Design review of the part built by this model. Coordinates are the model's own, in mm. A direction names the side the tool comes from. Give positions to 0.01 mm unless a question says otherwise; leave off trailing zeros. Loops run counter-clockwise (first coordinate to the right, second up) from the corner with the lowest first, then second, coordinate; pieces in that order, holes last. Notation, with made-up numbers: (34.5, -26.5) -> (55.5, -26.5) arc R35 ccw to (55.5, 5.5) -> close; hole circle Ø10 at (12, 6.25). An arc over 180 degrees is marked (long way). Answer in a Markdown table with one row per item. Add a question column.
(1) Draft analysis for pull direction X (two halves, no side actions). For faces 1 (the flat face through (-25, 1, 25)), 2 (the flat face through (19.104, 55.481, -0.675)), state which applies: +X half, -X half, draft (parallel to the pull), parting line (faces both ways), or undercut.
(2) For faces 3 (the cylindrical face through (2.994, 22.804, -0.084)), 4 (the flat face through (33, -49, -12)), 5 (the flat face through (-46.86, 35.31, -0.68)), list the 3-axis set-ups (+Z, -Z, +X, -X, +Y, -Y) from which the entire face can be reached by the end or side of a thin tool; tool diameter is ignored.
(3) Consider section C-C on x = -58.5. Write out the cut boundary in (y, z).
(4) For line 1 (Y direction, x = 0, z = -11); line 2 (Y direction, x = -59.5, z = -12.5); line 3 (X direction, y = 20, z = -10), list the stretches that pass through material, from the lowest coordinate up.
(5) Consider section D-D on y = -68. Write out the cut boundary in (x, z).
(6) For pin 1 (2 mm diameter, centred on y = 52, z = 18.5, fed in from +X); pin 2 (1.5 mm diameter, centred on x = 6.5, z = -3.5, fed in from -Y); pin 3 (24 mm diameter, centred on x = 7.5, y = 66.5, fed in from +Z); pin 4 (3 mm diameter, centred on x = 30, y = 0, fed in from +Z), all flat-tipped, find the tip position at first contact; note any pin that passes through.
(7) Consider section A-A on z = -18. Write out the cut boundary in (x, y), then the cut area to 3 significant figures.
from build123d import *
from build123d.topology import SkipClean

# Parameters (mm, degrees)
SKETCH1_R           = 90
BOSS_EXTRUDE1_DEPTH = 25
SKETCH3_R           = 24
CUT_EXTRUDE2_DEPTH  = 19
CUT_EXTRUDE3_START  = -19
SKETCH4_R           = 24
CUT_EXTRUDE3_DEPTH  = 19
SKETCH5_R           = 23
CUT_EXTRUDE4_DEPTH  = 12
SKETCH6_R           = 82
SKETCH6_R_2         = 36
CUT_EXTRUDE7_DEPTH  = 12
CUT_EXTRUDE8_START  = -12
SKETCH8_R           = 82
SKETCH8_R_2         = 36
CUT_EXTRUDE8_DEPTH  = 12
CUT_EXTRUDE10_START = -25
CUT_EXTRUDE10_DEPTH = 25
CUT_EXTRUDE11_DEPTH = 25
SKETCH13_R          = 2
CUT_EXTRUDE12_DEPTH = 137.747943312


with BuildPart() as part:
    # Sketch1 → Boss-Extrude1 (new, symmetric)
    with BuildSketch(Plane.XY):
        Circle(SKETCH1_R)
    extrude(amount=BOSS_EXTRUDE1_DEPTH, both=True)

    # Sketch3 → Cut-Extrude2 (cut)
    with BuildSketch(Plane.XY.offset(25)):
        Circle(SKETCH3_R)
    extrude(amount=-CUT_EXTRUDE2_DEPTH, mode=Mode.SUBTRACT)

    # Sketch4 → Cut-Extrude3 (cut)
    with BuildSketch(Plane(origin=(0, 0, -25), x_dir=(-1, 0, 0), z_dir=(0, 0, -1)).offset(CUT_EXTRUDE3_START)):
        with Locations(Location((0, 0, 0), (0, 0, 180))):
            Circle(SKETCH4_R)
    extrude(amount=CUT_EXTRUDE3_DEPTH, mode=Mode.SUBTRACT)

    # Sketch5 → Cut-Extrude4 (cut)
    with BuildSketch(Plane(origin=(0, 0, -6), x_dir=(-1, 0, 0), z_dir=(0, 0, -1))):
        Circle(SKETCH5_R)
    extrude(amount=-CUT_EXTRUDE4_DEPTH, mode=Mode.SUBTRACT)

    # Sketch6 → Cut-Extrude7 (cut)
    with BuildSketch(Plane(origin=(0, 0, -25), x_dir=(-1, 0, 0), z_dir=(0, 0, -1))):
        Circle(SKETCH6_R)
        Circle(SKETCH6_R_2, mode=Mode.SUBTRACT)
    extrude(amount=-CUT_EXTRUDE7_DEPTH, mode=Mode.SUBTRACT)

    # Sketch8 → Cut-Extrude8 (cut)
    with BuildSketch(Plane.XY.offset(25).offset(CUT_EXTRUDE8_START)):
        with Locations(Location((0, 0, 0), (0, 0, 180))):
            Circle(SKETCH8_R)
        with Locations(Location((0, 0, 0), (0, 0, 180))):
            Circle(SKETCH8_R_2, mode=Mode.SUBTRACT)
    extrude(amount=CUT_EXTRUDE8_DEPTH, mode=Mode.SUBTRACT)

    # Sketch11 → Cut-Extrude10 (cut)
    with SkipClean():  # the faces are left unmerged after this step: merging them gives an invalid solid
        with BuildSketch(Plane.XY.offset(13).offset(CUT_EXTRUDE10_START)):
            with BuildLine():
                Line((11.124611797, 34.238034587), (25.339393539, 77.986634336))
                ThreePointArc((25.339393539, 77.986634336), (0, 82), (-25.339393539, 77.986634336))
                Line((-25.339393539, 77.986634336), (-11.124611798, 34.238034587))
                ThreePointArc((-11.124611798, 34.238034587), (0, 36), (11.124611797, 34.238034587))
            make_face()
            with BuildLine():
                Line((29.124611798, 21.160269083), (66.339393539, 48.198390688))
                ThreePointArc((66.339393539, 48.198390688), (77.986634336, 25.339393539), (82, 0))
                Line((82, 0), (36, 0))
                ThreePointArc((36, 0), (34.238034587, 11.124611797), (29.124611798, 21.160269083))
            make_face()
            with BuildLine():
                Line((29.124611798, -21.160269083), (66.339393539, -48.198390688))
                ThreePointArc((66.339393539, -48.198390688), (48.198390688, -66.339393539), (25.339393539, -77.986634336))
                Line((25.339393539, -77.986634336), (11.124611797, -34.238034587))
                ThreePointArc((11.124611797, -34.238034587), (21.160269083, -29.124611798), (29.124611798, -21.160269083))
            make_face()
            with BuildLine():
                Line((-11.124611797, -34.238034587), (-25.339393539, -77.986634336))
                ThreePointArc((-25.339393539, -77.986634336), (-48.198390688, -66.339393539), (-66.339393539, -48.198390688))
                Line((-66.339393539, -48.198390688), (-29.124611798, -21.160269083))
                ThreePointArc((-29.124611798, -21.160269083), (-21.160269083, -29.124611798), (-11.124611797, -34.238034587))
            make_face()
            with BuildLine():
                Line((-36, 0), (-82, 0))
                ThreePointArc((-82, 0), (-77.986634336, 25.339393539), (-66.339393539, 48.198390688))
                Line((-66.339393539, 48.198390688), (-29.124611798, 21.160269083))
                ThreePointArc((-29.124611798, 21.160269083), (-34.238034587, 11.124611797), (-36, 0))
            make_face()
        extrude(amount=CUT_EXTRUDE10_DEPTH, mode=Mode.SUBTRACT)

    # Sketch12 → Cut-Extrude11 (cut)
    with SkipClean():  # the faces are left unmerged after this step: merging them gives an invalid solid
        with BuildSketch(Plane(origin=(0, 0, -13), x_dir=(-1, 0, 0), z_dir=(0, 0, -1))):
            with BuildLine():
                ThreePointArc((-28.750878362, 21.665340833), (-21.160269083, 29.124611797), (-11.72045356, 34.038668722))
                Line((-11.72045356, 34.038668722), (-26.696588665, 77.532523199))
                ThreePointArc((-26.696588665, 77.532523199), (-48.198390688, 66.339393539), (-65.488111824, 49.348831898))
                Line((-65.488111824, 49.348831898), (-28.750878362, 21.665340833))
            make_face()
            with BuildLine():
                Line((26.696588665, 77.532523199), (11.72045356, 34.038668722))
                ThreePointArc((11.72045356, 34.038668722), (21.160269083, 29.124611797), (28.750878362, 21.665340833))
                Line((28.750878362, 21.665340833), (65.488111824, 49.348831898))
                ThreePointArc((65.488111824, 49.348831898), (48.198390688, 66.339393539), (26.696588665, 77.532523199))
            make_face()
            with BuildLine():
                Line((81.987511003, -1.431097328), (35.994517026, -0.628286632))
                ThreePointArc((35.994517026, -0.628286632), (34.238034587, -11.124611797), (29.489473594, -20.648751709))
                Line((29.489473594, -20.648751709), (67.170467632, -47.033267781))
                ThreePointArc((67.170467632, -47.033267781), (77.986634336, -25.339393539), (81.987511003, -1.431097328))
            make_face()
            with BuildLine():
                ThreePointArc((-29.489473594, -20.648751709), (-34.238034587, -11.124611797), (-35.994517026, -0.628286632))
                Line((-35.994517026, -0.628286632), (-81.987511003, -1.431097328))
                ThreePointArc((-81.987511003, -1.431097328), (-77.986634336, -25.339393539), (-67.170467632, -47.033267781))
                Line((-67.170467632, -47.033267781), (-29.489473594, -20.648751709))
            make_face()
            with BuildLine():
                Line((23.974479787, -78.416989989), (10.52538137, -34.426971215))
                ThreePointArc((10.52538137, -34.426971215), (0, -36), (-10.52538137, -34.426971215))
                Line((-10.52538137, -34.426971215), (-23.974479787, -78.416989989))
                ThreePointArc((-23.974479787, -78.416989989), (0, -82), (23.974479787, -78.416989989))
            make_face()
        extrude(amount=-CUT_EXTRUDE11_DEPTH, mode=Mode.SUBTRACT)

    # Sketch13 → Cut-Extrude12 (cut, through all)
    with SkipClean():  # the faces are left unmerged after this step: merging them gives an invalid solid
        with BuildSketch(Plane(origin=(0, 0, -25), x_dir=(-1, 0, 0), z_dir=(0, 0, -1))):
            with Locations((0, 30)):
                Circle(SKETCH13_R)
            with Locations((30, 0)):
                Circle(SKETCH13_R)
            with Locations((0, -30)):
                Circle(SKETCH13_R)
            with Locations((-30, 0)):
                Circle(SKETCH13_R)
        extrude(amount=-CUT_EXTRUDE12_DEPTH, mode=Mode.SUBTRACT)


solid = part.part
Values follow:
| question | item | result |
|---|---|---|
| 1 | face 1 | draft |
| 1 | face 2 | undercut |
| 2 | face 3 | +Z, -Z |
| 2 | face 4 | +Z |
| 2 | face 5 | -Z |
| 3 | outline | (-68.39, -25) -> (-57.46, -25) -> (-57.46, -13) -> (-40.96, -13) -> (-40.96, 12) -> (-1.02, 12) -> (-1.02, -13) -> (44.08, -13) -> (44.08, 12) -> (57.46, 12) -> (57.46, -25) -> (68.39, -25) -> (68.39, 25) -> (57.46, 25) -> (57.46, 13) -> (42.5, 13) -> (42.5, -12) -> (0, -12) -> (0, 13) -> (-42.5, 13) -> (-42.5, -12) -> (-57.46, -12) -> (-57.46, 25) -> (-68.39, 25) -> close |
| 4 | line 1 | -90 to -82, -36 to -32, -28 to -24, 24 to 28, 32 to 36, 82 to 90 |
| 4 | line 2 | -67.53 to -41.66, -1.04 to 44.84, 56.42 to 67.53 |
| 4 | line 3 | -87.75 to -79.52, -29.93 to -13.27, 13.27 to 29.93, 79.52 to 87.75 |
| 5 | outline | (-58.96, -25) -> (-45.83, -25) -> (-45.83, -13) -> (-20.79, -13) -> (-20.79, 12) -> (20.79, 12) -> (20.79, -13) -> (45.83, -13) -> (45.83, -25) -> (58.96, -25) -> (58.96, 25) -> (45.83, 25) -> (45.83, -12) -> (22.09, -12) -> (22.09, 13) -> (-22.09, 13) -> (-22.09, -12) -> (-45.83, -12) -> (-45.83, 25) -> (-58.96, 25) -> close |
| 6 | pin 1 | x = 74.16 |
| 6 | pin 2 | y = -89.82 |
| 6 | pin 3 | z = -12 |
| 6 | pin 4 | through |
| 7 | outline | circle Ø180 at (0, 0); circle Ø72 at (0, 0); hole circle Ø164 at (0, 0); hole circle Ø4 at (-30, 0); hole circle Ø48 at (0, 0); hole circle Ø4 at (0, -30); hole circle Ø4 at (0, 30); hole circle Ø4 at (30, 0) |
| 7 | area | 6,530 mm2 |
